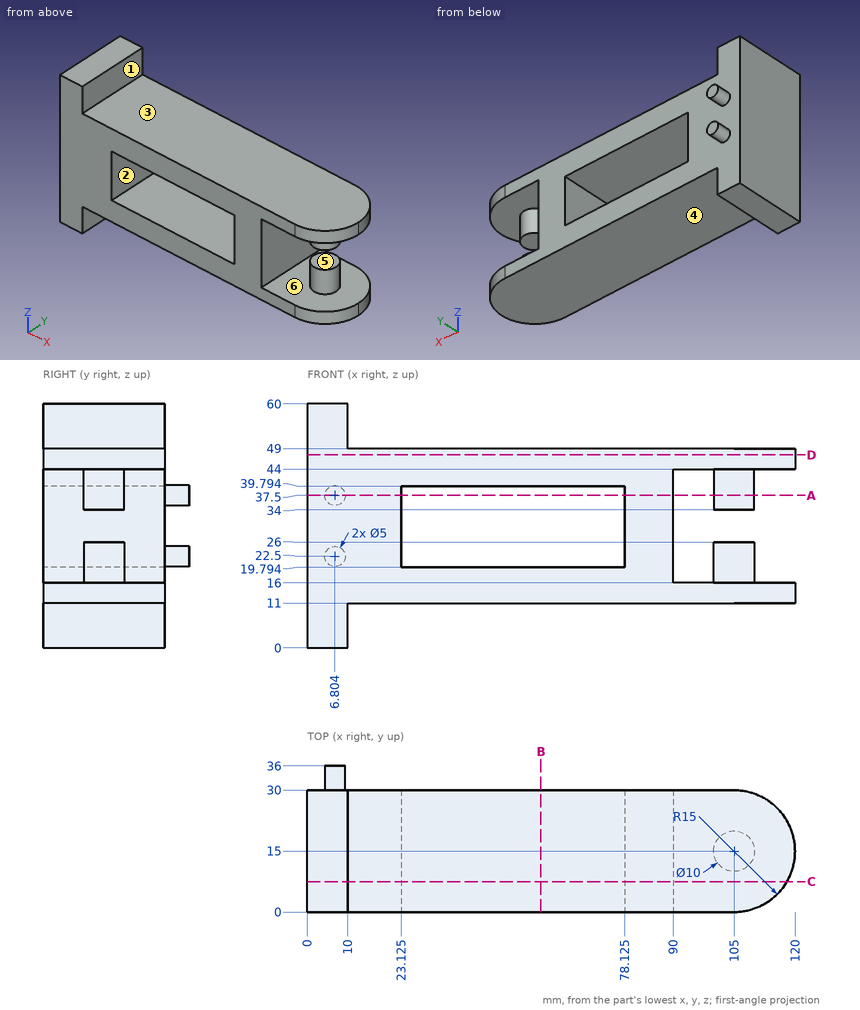
For this review, use the dimensioned drawing (mm, ordinates from the lowest corner) and the shaded views. A direction names the side the tool comes from. Round coordinates to 2 decimals unless told otherwise and drop trailing zeros. Loops run counter-clockwise (first coordinate to the right, second up) from the corner with the lowest first, then second, coordinate; pieces in that order, holes last. Notation, with made-up numbers: (16.5, 87) -> (58.5, 87) arc R24 cw to (58.5, 97) -> close; hole circle Ø8 at (70, -35.75). An arc over 180 degrees is marked (long way). Write item = value, one per line. Start each with the question number.
Item 1: Mouldability with a two-part tool opening along X and no side actions: class the marked faces 1, 2 and 3 as released by +X, released by -X, zero draft, split by the parting line, or undercut.
Item 2: Take a section at B-B on x = 57.5. Give the boundary of the cut face in (y, z).
Item 3: Take a section at D-D on z = 47.5. Give the boundary of the cut face in (x, y), plus the area to 3 significant figures.
Item 4: Take a section at C-C on y = 7.5. Give the boundary of the cut face in (x, z) (1 decimal), plus the area to 3 significant figures.
Item 5: Insertion check: pin 1 (14 mm diameter, centred on y = 21.5, z = 31, fed in from +X); pin 2 (1 mm diameter, centred on x = 74.5, y = 11.5, fed in from +Z); pin 3 (5 mm diameter, centred on x = 103, y = 14, fed in from -Z). Each pin has a flat end and moves straight along its axis. Give the tip position at first contact, or say it passes through.
Item 6: Take a section at A-A on z = 37.5. Give the boundary of the cut face in (x, y) (1 decimal).
Item 7: For the marked faces 4, 5 and 6, list the 3-axis set-ups (+Z, -Z, +X, -X, +Y, -Y) from which the entire face can be reached by the end or side of a thin tool; tool diameter is ignored.
Item 8: To check wall thickness, follow L1, parallel to X at y = 15.5, z = 37 (1 decimal); L2, parallel to Z at x = 47.5, y = 20; L3, parallel to Z at x = 108, y = 12.5. State the ranges of each line that lie inside material, in increasing order.
Result:
q1.face_1 = released by +X
q1.face_2 = undercut
q1.face_3 = zero draft
q2.outline = (0, 11) -> (30, 11) -> (30, 19.79) -> (0, 19.79) -> close; (0, 39.79) -> (30, 39.79) -> (30, 49) -> (0, 49) -> close
q3.outline = (0, 0) -> (105, 0) arc R15 ccw to (105, 30) -> (0, 30) -> close
q3.area = 3,500 mm²
q4.outline = (0, 0) -> (10, 0) -> (10, 11) -> (118, 11) -> (118, 16) -> (90, 16) -> (90, 44) -> (118, 44) -> (118, 49) -> (10, 49) -> (10, 60) -> (0, 60) -> close; hole (23.1, 19.8) -> (78.1, 19.8) -> (78.1, 39.8) -> (23.1, 39.8) -> close
q4.area = 2,820 mm²
q5.pin_1 = 110
q5.pin_2 = 49
q5.pin_3 = 11
q6.outline = (0, 0) -> (23.1, 0) -> (23.1, 30) -> (9.3, 30) -> (9.3, 36) -> (4.3, 36) -> (4.3, 30) -> (0, 30) -> close; (78.1, 0) -> (90, 0) -> (90, 30) -> (78.1, 30) -> close; circle Ø10 at (105, 15)
q7.face_4 = -Z, +X, +Y, -Y
q7.face_5 = +X, +Y, -Y
q7.face_6 = none
q8.L1 = 0 to 23.1, 78.1 to 90, 100 to 110
q8.L2 = 11 to 19.79, 39.79 to 49
q8.L3 = 11 to 26, 34 to 49
